from build123d import *

# Parameters (mm, degrees)
SKETCH022_R      = 8
EXTRUDE011_DEPTH = 150
EXTRUDE010_DEPTH = 30
SKETCH020_W      = 15
SKETCH020_H      = 79.05159
SKETCH020_H_2    = 80
EXTRUDE009_DEPTH = 150


with BuildPart() as extrude011:
    # Sketch022 → Extrude011 (new body, symmetric)
    with BuildSketch(Plane.YZ):
        Circle(SKETCH022_R)
    extrude(amount=EXTRUDE011_DEPTH, both=True)


with BuildPart() as extrude010:
    # Sketch021 → Extrude010 (new body, symmetric)
    with BuildSketch(Plane.XZ):
        with BuildLine():
            Line((38.5, 5), (38.5, -5))
            ThreePointArc((33.5, -10), (37.035534, -8.535534), (38.5, -5))
            Line((33.5, -10), (-33.5, -10))
            ThreePointArc((-38.5, -5), (-37.035534, -8.535534), (-33.5, -10))
            Line((-38.5, -5), (-38.5, 5))
            ThreePointArc((-33.5, 10), (-37.035534, 8.535534), (-38.5, 5))
            Line((-33.5, 10), (33.5, 10))
            ThreePointArc((38.5, 5), (37.035534, 8.535534), (33.5, 10))
        make_face()
    extrude(amount=EXTRUDE010_DEPTH, both=True)


with BuildPart() as extrude009:
    # Sketch020 → Extrude009 (new body, symmetric)
    with BuildSketch(Plane.YZ):
        with Locations((-21, 0.159191)):
            Rectangle(SKETCH020_W, SKETCH020_H)
        with Locations((21, -0.315014)):
            Rectangle(SKETCH020_W, SKETCH020_H_2)
    extrude(amount=EXTRUDE009_DEPTH, both=True)


with BuildPart() as obj1:
    # Sketch019 → Revolve001 (revolve)
    with BuildSketch(Plane.XZ):
        Polygon((-62.5, 0), (-62.5, 13.5), (-38.5, 18), (38.5, 18), (62.5, 13.5), (62.5, 0), align=None)
    revolve(axis=Axis((-62.5, 0, 0), (-1, 0, 0)))

    # Cut009: cut Extrude009
    add(extrude009.part, mode=Mode.SUBTRACT)

    # Cut010: cut Extrude010
    add(extrude010.part, mode=Mode.SUBTRACT)

    # Cut011: cut Extrude011
    add(extrude011.part, mode=Mode.SUBTRACT)


with BuildPart() as obj1_1:
    # Cut011 placement: moved
    add(obj1.part.moved(Location((-190, 0, 0))))


solid = obj1_1.part
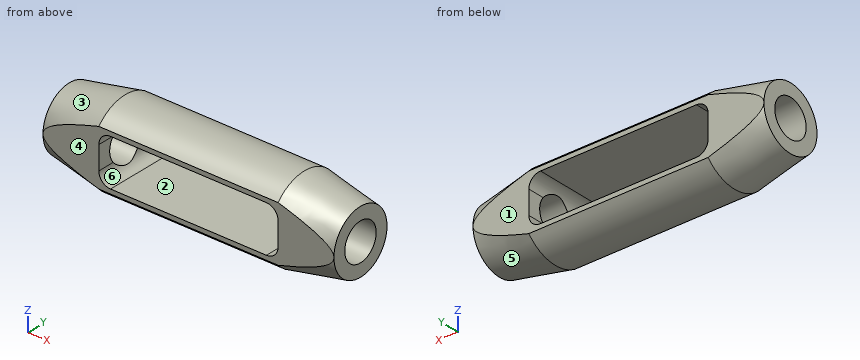
Check sheet for the modelled part. Datum: model origin and axes. Units: mm. Face numbers are marked on the shaded views. A direction names the side the tool comes from. Give positions to 0.01 mm unless a question says otherwise; leave off trailing zeros. Loops run counter-clockwise (first coordinate to the right, second up) from the corner with the lowest first, then second, coordinate; pieces in that order, holes last. Notation, with made-up numbers: M -24.5,71 L 0.5,71 A32 ccw 0.5,110 Z; hole C -38,59 d2. An arc over 180 degrees is marked long. Answer as a JSON object with one key per item and string values. Group by question number.
Q1. Cross-section at B-B on x = -194.5. Record the cut outline in (y, z).
Q2. Release check for a two-part mould opening along X. For the marked faces 3, 4, 5 and 6 record: released by +X, released by -X, zero draft, split by the parting line, or undercut.
Q3. Material ranges on line 1 along X through (y, z) = (-3, -8); line 2 along Z through (x, y) = (-219, -1.5); line 3 along X through (y, z) = (8.25, -4), recorded low to high. Write a range as [from, to].
Q4. Go/stop test with flat-tipped pins: P1, Ø13, axis at y = 0, z = 0, coming from the +X side; P2, Ø1.5, axis at x = -183, y = 3, coming from the +Z side; P3, Ø12, axis at x = -191, y = 5, coming from the -Z side; P4, Ø1, axis at x = -233.5, y = 2, coming from the -Z side. Record where each tip stops, or that it passes through.
Q5. Access from +Z, -Z, +X, -X, +Y, -Y to the whole of each face (thin tool, end or side, straight path). Record for the marked faces 1 and 2.
Q6. Cross-section at C-C on x = -146. Record the cut outline in (y, z), then the cut area to 3 significant figures.
Q7. Cross-section at D-D on z = -2. Give the number of separate pieces and of enclosed holes in the cut face, then the cut area to 3 significant figures.
Q8. Cross-section at A-A on y = 0. Record the cut outline in (x, z), then the cut area to 3 significant figures.
Evaluation:
{
 "1": {"outline": "M -13.5,-11.91 A18 ccw 13.5,-11.91 L 13.5,-10 L -13.5,-10 Z; M -13.5,10 L 13.5,10 L 13.5,11.91 A18 ccw -13.5,11.91 Z"},
 "2": {"face 3": "released by -X", "face 4": "zero draft", "face 5": "released by +X", "face 6": "undercut"},
 "3": {"line 1": "x = [-252.5, -227.5], [-152.5, -127.5]", "line 2": "z = [-17.94, -10], [10, 17.94]", "line 3": "x = [-252.5, -228.5], [-151.5, -127.5]"},
 "4": {"P1": "passes through", "P2": "stops at z = 17.86", "P3": "stops at z = -18", "P4": "stops at z = -17.05"},
 "5": {"face 1": "+Z, -Z, +X, -X, +Y", "face 2": "+Y, -Y"},
 "6": {"outline": "M -13.5,-10.28 A16.97 ccw 13.5,-10.28 L 13.5,10.28 A16.97 ccw -13.5,10.28 Z; hole C 0,0 d16", "area": "606 mm2"},
 "7": {"separate pieces": "4", "enclosed holes": "0", "area": "552 mm2"},
 "8": {"outline": "M -252.5,-13.5 L -228.5,-18 L -151.5,-18 L -127.5,-13.5 L -127.5,-8 L -152.5,-8 A5 cw -156.5,-10 L -223.5,-10 A5 cw -227.5,-8 L -252.5,-8 Z; M -252.5,8 L -227.5,8 A5 cw -223.5,10 L -156.5,10 A5 cw -152.5,8 L -127.5,8 L -127.5,13.5 L -151.5,18 L -228.5,18 L -252.5,13.5 Z", "area": "1,990 mm2"}
}
